Can you work these out from the drawing? Everything is in mm from the part's minimum corner. A direction names the side the tool comes from. Give positions to 0.01 mm unless a question says otherwise; leave off trailing zeros. Write each loop counter-clockwise with the first axis right and the second up, starting at its lowest first coordinate (ties: lowest second). Pieces come first, ordered by that corner, then holes. Notation, with made-up numbers: (66, -20) - (88, -20) arc R29 ccw to (88, 4) - close; hole circle Ø5 at (-15, 40). An arc over 180 degrees is marked (long way). Write each question's results on one line, items separated by ' | '. Start each with the question number.
Item 1: Suppose I cut it at D-D on z = 12. List the corners of the cut face in (x, y) for me.
Item 2: Suppose I cut it at A-A on z = 4. List the corners of the cut face in (x, y) for me.
Item 3: We'd pull the mould along Y, two halves only. Please class the marked faces 1, 2 and 3: +Y half, -Y half, draft (parallel to the pull), parting line (faces both ways), or undercut.
Item 4: Suppose I cut it at C-C on y = 23.25. List the corners of the cut face in (x, z) for me.
Item 5: Suppose I cut it at B-B on x = 3.5. List the corners of the cut face in (y, z) for me.
Item 6: Which directions (+Z, -Z, +X, -X, +Y, -Y) give clear straight access to the entire face, cutting with the end or side of a thin tool? Please do the marked faces 4, 5 and 6.
Item 7: Please list where these lines run through material, in increasing order: line 1 along X through (y, z) = (21, 22.75); line 2 along Y through (x, z) = (11.5, 22.5) (1 decimal); line 3 along Y through (x, z) = (9.25, 3.75).
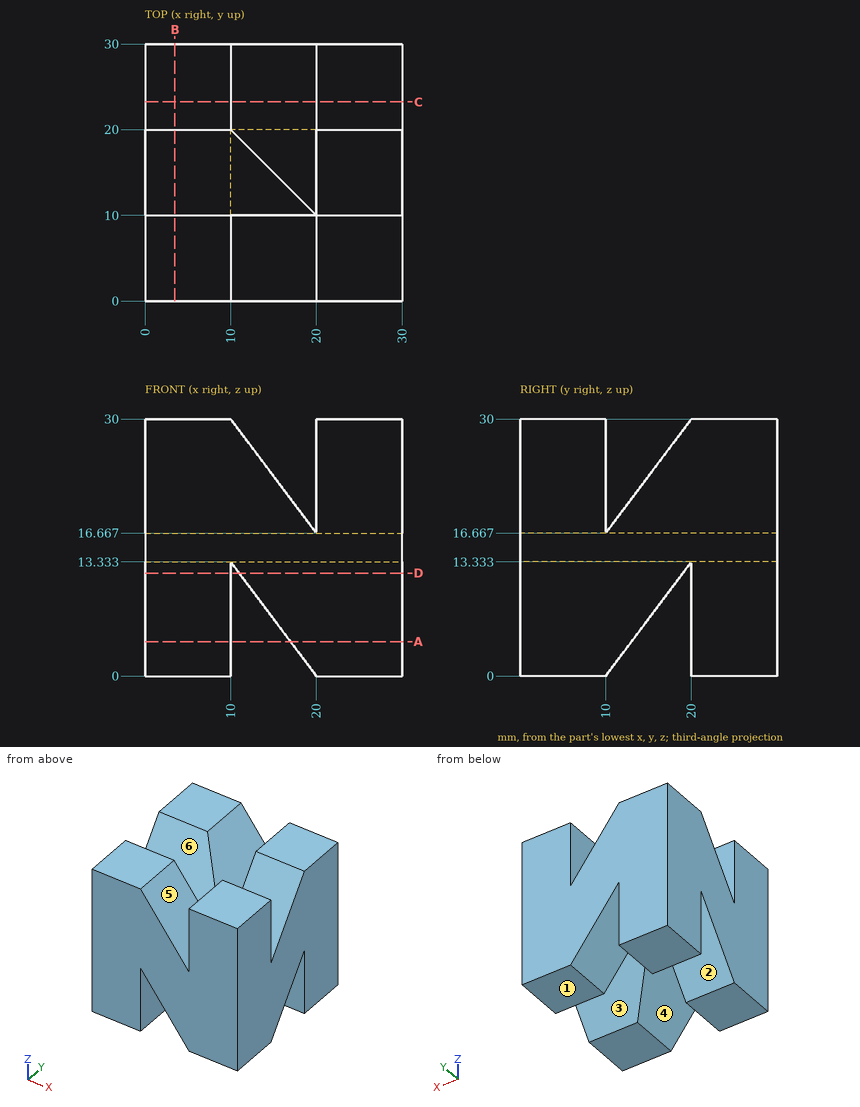
Checked values:
1) outline: (0, 0) - (10, 0) - (10, 19) - (0, 19) - close; (0, 20) - (10, 20) - (10, 30) - (0, 30) - close; (11, 0) - (30, 0) - (30, 19) - (11, 19) - close; (11, 20) - (30, 20) - (30, 30) - (11, 30) - close
2) outline: (0, 0) - (10, 0) - (10, 13) - (0, 13) - close; (0, 20) - (10, 20) - (10, 30) - (0, 30) - close; (17, 0) - (30, 0) - (30, 13) - (17, 13) - close; (17, 20) - (30, 20) - (30, 30) - (17, 30) - close
3) face 1: draft | face 2: undercut | face 3: undercut
4) outline: (0, 0) - (10, 0) - (10, 13.33) - (20, 0) - (30, 0) - (30, 30) - (20, 30) - (20, 16.67) - (10, 30) - (0, 30) - close
5) outline: (0, 0) - (10, 0) - (20, 13.33) - (20, 0) - (30, 0) - (30, 30) - (20, 30) - (10, 16.67) - (10, 30) - (0, 30) - close
6) face 4: -Z, +Y, -Y | face 5: +Z, +Y, -Y | face 6: +Z, +X, -X
7) line 1: x = 0 to 15.44, 20 to 30 | line 2: y = 0 to 10, 14.4 to 30 | line 3: y = 0 to 12.81, 20 to 30
